Autodesk Inventor part; units mm, degrees
ref_plane "YZ Plane" through (0, 0, 0) normal (1, 0, 0) x (0, 1, 0)
ref_plane "XZ Plane" through (0, 0, 0) normal (0, 1, 0) x (-1, 0, 0)
ref_plane "XY Plane" through (0, 0, 0) normal (0, 0, 1) x (1, 0, 0)
sketch "Sketch1" plane through (0, 0, 0) normal (0, 0, 1) x (1, 0, 0)
  line L0 (-10.6066, 0) -> (0, 10.6066)
  line L1 (0, 10.6066) -> (10.6066, 0)
  line L2 (10.6066, 0) -> (0, -10.6066)
  line L3 (0, -10.6066) -> (-10.6066, 0)
  arc A0 (-25.9808, -15) -> (25.9808, -15) centre (0, 0) ccw
  line L4 (118.3568, 145) -> (-118.3568, 145)
  line L5 (7.5, 35.6066) -> (13.85, 35.6066)
  line L6 (13.85, 35.6066) -> (13.85, 15.6066)
  line L7 (13.85, 15.6066) -> (7.5, 15.6066)
  line L8 (7.5, 15.6066) -> (7.5, 35.6066)
  line L9 (-5, 43.1066) -> (5, 43.1066)
  line L10 (5, 43.1066) -> (5, 13.1066)
  line L11 (5, 13.1066) -> (-5, 13.1066)
  line L12 (-5, 13.1066) -> (-5, 43.1066)
  line L13 (118.3568, 145) -> (25.9808, -15)
  line L14 (-25.9808, -15) -> (-118.3568, 145)
  point P0 (0, 13.1066)
  dimension "d0" = 15
  dimension "d4" = 30
  dimension "d6" = 6.35
  dimension "d7" = 20
  dimension "d8" = 5
  dimension "d16" = 10
  dimension "d17" = 2.5
  dimension "d18" = 2.5
  dimension "d19" = 30
  dimension "d23" = 60
  dimension "d24" = 175
extrude "Extrusion1" add sketch "Sketch1" along normal blind 6.35
properties part number "Frame_Lower_Plate_Top"
Check sheet for the modelled part. Datum: model origin and axes. Units: mm. A direction names the side the tool comes from. Coordinates: 2 decimals unless noted, no trailing zeros. Loops run counter-clockwise (first coordinate to the right, second up) from the corner with the lowest first, then second, coordinate; pieces in that order, holes last.
1) Sectioned sample at A-A (z = 1.25). Record the boundary of the cut face in (x, y), and give its area (3 significant figures).
2) Sectioned sample at C-C (x = -99). Record the boundary of the cut face in (y, z), and give its area (3 significant figures).
3) Sectioned sample at D-D (y = 127). Record the boundary of the cut face in (x, z).
4) Gauge pin test, flat ends, axial feed: pin 1 (2 mm diameter, centred on y = 19.5, z = 3.5, fed in from -X); pin 2 (1 mm diameter, centred on x = 47, z = 0.5, fed in from -Y); pin 3 (1.5 mm diameter, centred on x = -21, z = 3, fed in from -Y). Record the tip position at first contact, or that the pin passes through.
5) Access from +Z, -Z, +X, -X, +Y, -Y to the whole of each face (thin tool, end or side, straight path). Record for faces 4 (the face through (-2, 78, 6.35)), 5 (the face through (5.229, 5.378, 3.131)).
6) Material ranges on probe 1 along X at (y, z) = (28, 3.25); probe 2 along X at (y, z) = (25.5, 1); probe 3 along Y at (x, z) = (-1.5, 6), recorded low to high.
7) Sectioned sample at B-B (y = -5.5). Record the boundary of the cut face in (x, z).
8) Release check for a two-part mould opening along X. For faces 1 (the face through (0, 43.107, 3)), 2 (the face through (-71.52, 63.88, 3.13)), 3 (the face through (0, -30, 3)) record: released by +X, released by -X, zero draft, split by the parting line, or undercut.
Check sheet entries:
1. outline: (-118.36, 145) - (-25.98, -15) arc R30 ccw to (25.98, -15) - (118.36, 145) - close; hole (-10.61, 0) - (0, -10.61) - (10.61, 0) - (0, 10.61) - close; hole (-5, 13.11) - (5, 13.11) - (5, 43.11) - (-5, 43.11) - close; hole (7.5, 15.61) - (13.85, 15.61) - (13.85, 35.61) - (7.5, 35.61) - close
1. area: 23,000 mm2
2. outline: (111.47, 0) - (145, 0) - (145, 6.35) - (111.47, 6.35) - close
2. area: 213 mm2
3. outline: (-107.96, 0) - (107.96, 0) - (107.96, 6.35) - (-107.96, 6.35) - close
4. pin 1: stops at x = -46.48
4. pin 2: stops at y = 20.54
4. pin 3: stops at y = -22.13
5. face 4: +Z, +X, -X, +Y, -Y
5. face 5: +Z, -Z
6. probe 1: x = -50.81 to -5, 5 to 7.5, 13.85 to 50.81
6. probe 2: x = -49.36 to -5, 5 to 7.5, 13.85 to 49.36
6. probe 3: y = -29.96 to -9.11, 9.11 to 13.11, 43.11 to 145
7. outline: (-31.47, 0) - (-5.11, 0) - (-5.11, 6.35) - (-31.47, 6.35) - close; (5.11, 0) - (31.47, 0) - (31.47, 6.35) - (5.11, 6.35) - close
8. face 1: undercut
8. face 2: released by -X
8. face 3: split by the parting line
